```python
from build123d import *

# Parameters (mm, degrees)
SKETCH2_R           = 2.25
BOSS_EXTRUDE1_DEPTH = 250


with BuildPart() as part:
    # Sketch2 → Boss-Extrude1 (new body)
    with BuildSketch(Plane(origin=(0, 0, 0), x_dir=(1, 0, 0), z_dir=(0, 1, 0))):
        with BuildLine():
            Line((-22.025, -12.575), (-22.025, 0.975))
            ThreePointArc((-22.025, 0.975), (-21.439213562, 2.389213562), (-20.025, 2.975))
            Line((-20.025, 2.975), (20.025, 2.975))
            ThreePointArc((20.025, 2.975), (21.439213562, 2.389213562), (22.025, 0.975))
            Line((22.025, 0.975), (22.025, -12.575))
            Line((22.025, -12.575), (29.925, -12.575))
            Line((29.925, -12.575), (29.925, 7.575))
            ThreePointArc((29.925, 7.575), (28.460533906, 11.110533906), (24.925, 12.575))
            Line((24.925, 12.575), (-24.925, 12.575))
            ThreePointArc((-24.925, 12.575), (-28.460533906, 11.110533906), (-29.925, 7.575))
            Line((-29.925, 7.575), (-29.925, -12.575))
            Line((-29.925, -12.575), (-22.025, -12.575))
        make_face()
        with Locations(Location((18.1, 8.575, 0), (0, 0, 270))):
            Circle(SKETCH2_R, mode=Mode.SUBTRACT)
        with Locations(Location((25.975, -8.825, 0), (0, 0, 270))):
            Circle(SKETCH2_R, mode=Mode.SUBTRACT)
        with Locations(Location((-25.975, -8.825, 0), (0, 0, 90))):
            Circle(SKETCH2_R, mode=Mode.SUBTRACT)
        with Locations(Location((-18.1, 8.575, 0), (0, 0, 90))):
            Circle(SKETCH2_R, mode=Mode.SUBTRACT)
    extrude(amount=-BOSS_EXTRUDE1_DEPTH)


solid = part.part
```
CAD build for the part. Positions are in the model's coordinates, mm. A direction names the side the tool comes from. Give positions to 0.01 mm unless a question says otherwise; leave off trailing zeros. Order: outer loops, then holes, each group sorted by start corner. A loop starts at its lowest first (then second) coordinate and runs counter-clockwise, first axis right, second up.
(1) Saw through at C-C, the plane x = 5.5. Give the cut face in (y, z) (3 decimals).
(2) Drill centre lines: L1, parallel to X at y = -113.5, z = -8.25; L2, parallel to X at y = -130.5, z = 8.5 (3 decimals); L3, parallel to Z at x = 25.5, y = -73 (3 decimals). Where is each one in solid material? Low to high.
(3) Flat gauge pins, fed straight in: pin 1 (5 mm diameter, centred on x = -10, y = -192, fed in from +Z) (3 decimals); pin 2 (4 mm diameter, centred on x = -18.1, z = -8.575, fed in from -Y). Where does each tip first touch, or does it go through?
(4) Saw through at A-A, the plane z = 3.5. Give the cut face in (x, y) (3 decimals), then the cut area to 3 significant figures.
(5) Tool access for faces 1 (the flat face through (0, -123, -2.975)), 2 (the flat face through (26, -123, 12.575)): list every direction of +Z, -Z, +X, -X, +Y, -Y with a clear straight run to the whole face (end or side of a thin tool).
(6) Mould opens along Z. For faces 3 (the flat face through (-29.925, -123, 2)), 4 (the flat face through (0, -123, -12.575)), 5 (the cylindrical face through (20, -123.25, -7.37)) say: released by +Z, released by -Z, zero draft, split by the parting line, or undercut.
(7) Saw through at B-B, the plane y = -192. Give the cut face in (x, z) (3 decimals), then the cut area to 3 significant figures.
Results found:
1. outline: (-250, -12.575) - (0, -12.575) - (0, -2.975) - (-250, -2.975) - close
2. L1: x = -29.88 to -20.33, -15.87 to 15.87, 20.33 to 29.88
2. L2: x = -29.925 to -28.201, -23.749 to -22.025, 22.025 to 23.749, 28.201 to 29.925
2. L3: z = -12.542 to 6.626, 11.024 to 12.575
3. pin 1: stops at z = -2.975
3. pin 2: passes through
4. outline: (-29.925, -250) - (-22.025, -250) - (-22.025, 0) - (-29.925, 0) - close; (22.025, -250) - (29.925, -250) - (29.925, 0) - (22.025, 0) - close
4. area: 3,950 mm2
5. face 1: +Z, +Y, -Y
5. face 2: +Z, +X, -X, +Y, -Y
6. face 3: zero draft
6. face 4: released by -Z
6. face 5: undercut
7. outline: (-29.925, -7.575) arc R5 ccw to (-24.925, -12.575) - (24.925, -12.575) arc R5 ccw to (29.925, -7.575) - (29.925, 12.575) - (22.025, 12.575) - (22.025, -0.975) arc R2 cw to (20.025, -2.975) - (-20.025, -2.975) arc R2 cw to (-22.025, -0.975) - (-22.025, 12.575) - (-29.925, 12.575) - close; hole circle Ø4.5 at (-25.975, 8.825); hole circle Ø4.5 at (-18.1, -8.575); hole circle Ø4.5 at (18.1, -8.575); hole circle Ø4.5 at (25.975, 8.825)
7. area: 748 mm2
